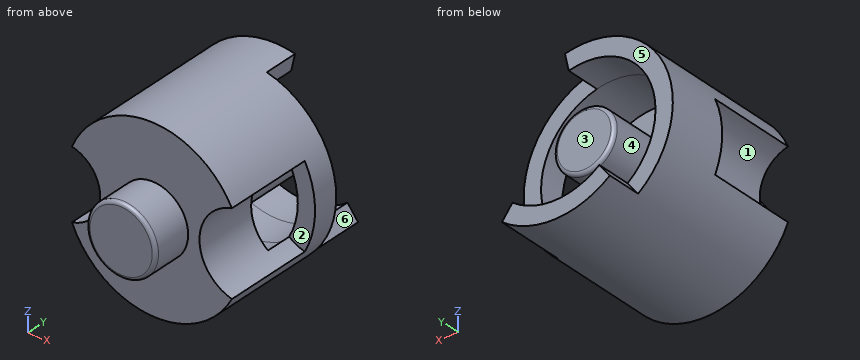
from build123d import *

# Parameters (mm, degrees)
SKETCH1_R           = 6.50875
BOSS_EXTRUDE1_DEPTH = 13.5382
SKETCH2_R           = 2.54
BOSS_EXTRUDE2_DEPTH = 2.921
CUT_EXTRUDE1_START  = -2.54
CUT_EXTRUDE1_DEPTH  = 2.54
CUT_EXTRUDE2_START  = -2.54
SKETCH4_R           = 2.2225
CUT_EXTRUDE2_DEPTH  = 2.54
CUT_EXTRUDE3_START  = -3.81
SKETCH5_R           = 5.23875
SKETCH5_R_2         = 2.2225
CUT_EXTRUDE3_DEPTH  = 3.81
CUT_EXTRUDE4_DEPTH  = 6.5532


with BuildPart() as part:
    # Sketch1 → Boss-Extrude1 (new body)
    with BuildSketch(Plane(origin=(0, 0, 0), x_dir=(1, 0, 0), z_dir=(0, 1, 0))):
        with Locations(Location((0, 0, 0), (0, 0, 270))):
            Circle(SKETCH1_R)
    extrude(amount=BOSS_EXTRUDE1_DEPTH)

    # Sketch2 → Boss-Extrude2 (add)
    with BuildSketch(Plane.XZ):
        with Locations(Location((0, 0, 0), (0, 0, 270))):
            Circle(SKETCH2_R)
    extrude(amount=BOSS_EXTRUDE2_DEPTH)

    # Sketch3 → Cut-Extrude1 (cut)
    with BuildSketch(Plane(origin=(0, 13.5382, 0), x_dir=(1, 0, 0), z_dir=(0, 1, 0)).offset(CUT_EXTRUDE1_START)):
        with BuildLine():
            Line((-3.189148936, 4.156179811), (-3.962275951, 5.163738554))
            ThreePointArc((-3.962275951, 5.163738554), (0, -6.50875), (3.962275951, 5.163738554))
            Line((3.962275951, 5.163738554), (3.189148936, 4.156179811))
            ThreePointArc((3.189148936, 4.156179811), (0, 5.23875), (-3.189148936, 4.156179811))
        make_face()
    extrude(amount=CUT_EXTRUDE1_DEPTH, mode=Mode.SUBTRACT)

    # Sketch4 → Cut-Extrude2 (cut)
    with BuildSketch(Plane(origin=(0, 10.9982, 0), x_dir=(1, 0, 0), z_dir=(0, 1, 0)).offset(CUT_EXTRUDE2_START)):
        with BuildLine():
            Line((3.962275951, 5.163738554), (3.189148936, 4.156179811))
            ThreePointArc((3.189148936, 4.156179811), (-5.114570707, 1.133873028), (1.133873028, -5.114570707))
            Line((1.133873028, -5.114570707), (1.408751337, -6.354466636))
            ThreePointArc((1.408751337, -6.354466636), (6.354466636, -1.408751337), (3.962275951, 5.163738554))
        make_face()
        with Locations(Location((0, 0, 0), (0, 0, 270))):
            Circle(SKETCH4_R, mode=Mode.SUBTRACT)
    extrude(amount=CUT_EXTRUDE2_DEPTH, mode=Mode.SUBTRACT)

    # Sketch5 → Cut-Extrude3 (cut)
    with BuildSketch(Plane(origin=(0, 8.4582, 0), x_dir=(1, 0, 0), z_dir=(0, 1, 0)).offset(CUT_EXTRUDE3_START)):
        with Locations(Location((0, 0, 0), (0, 0, 270))):
            Circle(SKETCH5_R)
        with Locations(Location((0, 0, 0), (0, 0, 270))):
            Circle(SKETCH5_R_2, mode=Mode.SUBTRACT)
    extrude(amount=CUT_EXTRUDE3_DEPTH, mode=Mode.SUBTRACT)

    # Sketch6 → Cut-Extrude4 (cut)
    with BuildSketch(Plane.XZ):
        with BuildLine():
            ThreePointArc((5.750958404, 3.048), (3.367961548, 0), (5.750958404, -3.048))
            ThreePointArc((5.750958404, -3.048), (6.50875, 0), (5.750958404, 3.048))
        make_face()
        with BuildLine():
            ThreePointArc((-5.992681083, 2.54), (-3.916853566, 0), (-5.992681083, -2.54))
            ThreePointArc((-5.992681083, -2.54), (-6.50875, 0), (-5.992681083, 2.54))
        make_face()
    extrude(amount=-CUT_EXTRUDE4_DEPTH, mode=Mode.SUBTRACT)

    # Fillet2: read off the stored shape, not the designer's step
    # Fillet2 outline → Fillet2 (revolve, cut)
    with BuildSketch(Plane.XY):
        with BuildLine():
            ThreePointArc((1.9685, 10.9982), (2.148105122, 10.923805122), (2.2225, 10.7442))
            Line((2.2225, 10.7442), (2.2225, 10.9982))
            Line((2.2225, 10.9982), (1.9685, 10.9982))
        make_face()
        with BuildLine():
            Line((2.54, -2.921), (2.54, -2.667))
            ThreePointArc((2.54, -2.667), (2.465605122, -2.846605122), (2.286, -2.921))
            Line((2.286, -2.921), (2.54, -2.921))
        make_face()
    revolve(axis=Axis((0, 0, 0), (0, 1, 0)), mode=Mode.SUBTRACT)

    # Fillet2 2 outline → Fillet2 2 (revolve)
    with BuildSketch(Plane.XY):
        with BuildLine():
            Line((2.2225, 4.9022), (2.2225, 4.6482))
            Line((2.2225, 4.6482), (2.4765, 4.6482))
            ThreePointArc((2.4765, 4.6482), (2.296894878, 4.722594878), (2.2225, 4.9022))
        make_face()
    revolve(axis=Axis((0, 0, 0), (0, 1, 0)))


solid = part.part
For this review, take the finished solid that the model builds, in its own axes (mm). Face numbers are marked on the shaded views. A direction names the side the tool comes from. Coordinates: 2 decimals unless noted, no trailing zeros. Order: outer loops, then holes, each group sorted by start corner. A loop starts at its lowest first (then second) coordinate and runs counter-clockwise, first axis right, second up. Notation, with made-up numbers: (23, 45) -> (45, 45) arc R34 ccw to (45, 76) -> close; hole circle Ø3 at (-13.75, -12). An arc over 180 degrees is marked (long way). Return JSON: item names as keys, results as strings.
1. The part is to be moulded in two halves that separate along X. For the marked faces 4, 5 and 6, say which applies: +X half, -X half, draft (parallel to the pull), parting line (faces both ways), or undercut.
Answer block:
{"face 4": "undercut", "face 5": "draft", "face 6": "+X half"}
2. We need section D-D on y = 5.25. Write out the cut boundary in (x, z) (1 decimal).
Answer block:
{"outline": "(-6, -2.5) arc R6.5 ccw to (5.8, -3) arc R3.1 cw to (4.6, -2.5) arc R5.2 cw to (-4.8, -2) arc R2.6 cw to start; (-6, 2.5) arc R2.6 cw to (-4.8, 2) arc R5.2 cw to (4.6, 2.5) arc R3.1 cw to (5.8, 3) arc R6.5 ccw to start; circle Ø4.4 at (0, 0)"}
3. Machinability: for the marked faces 1, 2 and 3, which of the approach directions +Z, -Z, +X, -X, +Y, -Y give a long, thin tool a straight path to every point of the face, cutting with its end or side? Answer none if there is none.
Answer block:
{"face 1": "-X, -Y", "face 2": "+X, -Y", "face 3": "+Z, +X, -X, +Y"}
4. We need section B-B on y = 10.25. Write out the cut boundary in (x, z) (1 decimal), and give its area (3 significant figures).
Answer block:
{"outline": "circle Ø4.4 at (0, 0); (1.1, 5.1) -> (1.4, 6.4) arc R6.5 ccw (long way) to (4, -5.2) -> (3.2, -4.2) arc R5.2 cw (long way) to start", "area": "45.5 mm²"}
5. We need section A-A on z = 0. Write out the cut boundary in (x, y), and give its area (3 significant figures).
Answer block:
{"outline": "(-6.51, 6.55) -> (-5.24, 6.55) -> (-5.24, 11) -> (-6.51, 11) -> close; (-3.92, 0) -> (-2.54, 0) -> (-2.54, -2.67) arc R0.25 ccw to (-2.29, -2.92) -> (2.29, -2.92) arc R0.25 ccw to (2.54, -2.67) -> (2.54, 0) -> (3.37, 0) -> (3.37, 4.65) -> (2.48, 4.65) arc R0.25 cw to (2.22, 4.9) -> (2.22, 10.74) arc R0.25 ccw to (1.97, 11) -> (-1.97, 11) arc R0.25 ccw to (-2.22, 10.74) -> (-2.22, 4.9) arc R0.25 cw to (-2.48, 4.65) -> (-3.92, 4.65) -> close; (5.24, 6.55) -> (6.51, 6.55) -> (6.51, 8.46) -> (5.24, 8.46) -> close", "area": "85.0 mm²"}
6. For pin 1 Ø2.5 at (x, z) = (-1.5, -1) entering from +Y; pin 2 Ø1 at (x, y) = (4.5, 9) entering from -Z; pin 3 Ø5 at (x, y) = (4, 3) entering from +Z; pin 4 Ø1.5 at (x, z) = (5.5, 0) entering from -Y, all flat-tipped, find the tip position at first contact; note any pin that passes through.
Answer block:
{"pin 1": "y = 11", "pin 2": "through", "pin 3": "z = 6.33", "pin 4": "y = 6.55"}
7. We need section C-C on x = 0. Write out the cut boundary in (y, z), and give its area (3 significant figures).
Answer block:
{"outline": "(-2.92, -2.29) arc R0.25 ccw to (-2.67, -2.54) -> (0, -2.54) -> (0, -6.51) -> (13.54, -6.51) -> (13.54, -5.24) -> (4.65, -5.24) -> (4.65, -2.48) arc R0.25 cw to (4.9, -2.22) -> (10.74, -2.22) arc R0.25 ccw to (11, -1.97) -> (11, 1.97) arc R0.25 ccw to (10.74, 2.22) -> (4.9, 2.22) arc R0.25 cw to (4.65, 2.48) -> (4.65, 5.24) -> (11, 5.24) -> (11, 6.51) -> (0, 6.51) -> (0, 2.54) -> (-2.67, 2.54) arc R0.25 ccw to (-2.92, 2.29) -> close", "area": "123 mm²"}
8. For line 1 (Z direction, x = 0, y = 7); line 2 (X direction, y = 10.1, z = 0), list the stretches that pass through material, from the lowest coordinate up. Write a range as from..to.
Answer block:
{"line 1": "-6.51..-5.24, -2.22..2.22, 5.24..6.51", "line 2": "-6.51..-5.24, -2.22..2.22"}
